Source: CAD feature listing. Evaluate the final solid. Frame: model axes, mm. A direction names the side the tool comes from. Give positions to 0.01 mm unless a question says otherwise; leave off trailing zeros. Loops run counter-clockwise (first coordinate to the right, second up) from the corner with the lowest first, then second, coordinate; pieces in that order, holes last. Notation, with made-up numbers: (42, 89.25) - (68, 89.25) arc R21 cw to (68, 128.25) - close; hole circle Ø4 at (88.5, 78.5). An arc over 180 degrees is marked (long way). Put each result on its own line as item: value.
```python
from build123d import *

# Parameters (mm, degrees)
SKETCH_1_W                = 90
SKETCH_1_H                = 150
EXTRUDE_1_DEPTH           = 5
SKETCH_4_R                = 36
CUT_EXTRUDE_1_DEPTH       = 89.034084308
HOLE_WIZARD_3_D           = 6.6
HOLE_WIZARD_3_CBORE_D     = 11
HOLE_WIZARD_3_CBORE_DEPTH = 6.8
HOLE_START                = -1.8
HOLE_WIZARD_2_DEPTH       = 6.8
HOLE_START_2              = -5
HOLE_WIZARD_2_2_DEPTH     = 3.2
CHAMFER_1_SIZE            = 12


# Read off the part's stored shape, not the designer's step: 打孔尺寸(%根据)内六角圆柱头螺钉的类型2
with BuildPart() as part:
    # 草图1 → 凸台-拉伸1 (new, symmetric)
    with BuildSketch(Plane.XY):
        Rectangle(SKETCH_1_W, SKETCH_1_H)
    extrude(amount=EXTRUDE_1_DEPTH, both=True)

    # 草图4 → 切除-拉伸1 (cut, through all)
    with BuildSketch(Plane.XY.offset(5)):
        Circle(SKETCH_4_R)
    extrude(amount=-CUT_EXTRUDE_1_DEPTH, mode=Mode.SUBTRACT)

    # 打孔尺寸(%根据)内六角圆柱头螺钉的类型3 (through all)
    with Locations(Plane(origin=(-31.75, 31.75, 5), x_dir=(1, 0, 0), z_dir=(0, 0, 1))):
        with Locations((0, 0), (63.5, 0), (0, -63.5), (63.5, -63.5)):
            CounterBoreHole(HOLE_WIZARD_3_D / 2, HOLE_WIZARD_3_CBORE_D / 2, HOLE_WIZARD_3_CBORE_DEPTH)

    # 打孔尺寸(%根据)内六角圆柱头螺钉的类型2 outline → 打孔尺寸(%根据)内六角圆柱头螺钉的类型2 (cut)
    with BuildSketch(Plane.XY.offset(HOLE_START)):
        with BuildLine():
            Line((-34, 59.5), (-26, 59.5))
            ThreePointArc((-26, 59.5), (-20.5, 65), (-26, 70.5))
            Line((-26, 70.5), (-34, 70.5))
            ThreePointArc((-34, 70.5), (-39.5, 65), (-34, 59.5))
        make_face()
        with BuildLine():
            ThreePointArc((34, 59.5), (39.5, 65), (34, 70.5))
            Line((34, 70.5), (26, 70.5))
            ThreePointArc((26, 70.5), (20.5, 65), (26, 59.5))
            Line((26, 59.5), (34, 59.5))
        make_face()
        with BuildLine():
            Line((-34, -70.5), (-26, -70.5))
            ThreePointArc((-26, -70.5), (-20.5, -65), (-26, -59.5))
            Line((-26, -59.5), (-34, -59.5))
            ThreePointArc((-34, -59.5), (-39.5, -65), (-34, -70.5))
        make_face()
        with BuildLine():
            ThreePointArc((34, -70.5), (39.5, -65), (34, -59.5))
            Line((34, -59.5), (26, -59.5))
            ThreePointArc((26, -59.5), (20.5, -65), (26, -70.5))
            Line((26, -70.5), (34, -70.5))
        make_face()
    extrude(amount=HOLE_WIZARD_2_DEPTH, mode=Mode.SUBTRACT)

    # Hole Wizard 2 2 outline → Hole Wizard 2 2 (cut)
    with BuildSketch(Plane.XY.offset(HOLE_START_2)):
        with BuildLine():
            Line((-34, 61.7), (-26, 61.7))
            ThreePointArc((-26, 61.7), (-22.7, 65), (-26, 68.3))
            Line((-26, 68.3), (-34, 68.3))
            ThreePointArc((-34, 68.3), (-37.3, 65), (-34, 61.7))
        make_face()
        with BuildLine():
            ThreePointArc((34, 61.7), (37.3, 65), (34, 68.3))
            Line((34, 68.3), (26, 68.3))
            ThreePointArc((26, 68.3), (22.7, 65), (26, 61.7))
            Line((26, 61.7), (34, 61.7))
        make_face()
        with BuildLine():
            Line((-34, -68.3), (-26, -68.3))
            ThreePointArc((-26, -68.3), (-22.7, -65), (-26, -61.7))
            Line((-26, -61.7), (-34, -61.7))
            ThreePointArc((-34, -61.7), (-37.3, -65), (-34, -68.3))
        make_face()
        with BuildLine():
            ThreePointArc((34, -68.3), (37.3, -65), (34, -61.7))
            Line((34, -61.7), (26, -61.7))
            ThreePointArc((26, -61.7), (22.7, -65), (26, -68.3))
            Line((26, -68.3), (34, -68.3))
        make_face()
    extrude(amount=HOLE_WIZARD_2_2_DEPTH, mode=Mode.SUBTRACT)

    # 倒角1
    chamfer_1_edges = [part.edges().sort_by_distance(p)[0] for p in [
        (45, -75, 0),
        (-45, -75, 0),
        (-45, 75, 0),
        (45, 75, 0),
    ]]
    chamfer(chamfer_1_edges, length=CHAMFER_1_SIZE)


solid = part.part
```
1) Mould query, pull axis X, two halves, no side actions, for faces 4 (the flat face through (19, -32, -5)), 5 (the cylindrical face through (31, 37.2, 1.6)). Classes: pulls with the +X half, pulls with the -X half, needs draft (parallel to the pull), parting line crosses it, or undercut.
Check result:
face 4: needs draft
face 5: undercut
2) Section query C-C, the plane z = -3.5. State how many separate pieces and enclosed holes the cut face has, plus the area to 3 significant figures.
Check result:
separate pieces: 1
enclosed holes: 9
area: 8,660 mm²
3) Section query A-A, the plane y = 0. Output: boundary loops of the cut face in (x, z), plus the area to 3 significant figures.
Check result:
outline: (-45, -5) - (-36, -5) - (-36, 5) - (-45, 5) - close; (36, -5) - (45, -5) - (45, 5) - (36, 5) - close
area: 180 mm²
4) Material intervals for line 1 along Y through (x, z) = (23, 2); line 2 along X through (y, z) = (-30, -2); line 3 along Y through (x, z) = (-23, -4), sorted ascending. Write a range as [from, to].
Check result:
line 1: [-75, -69.61], [-60.39, -27.69], [27.69, 60.39], [69.61, 75]
line 2: [-45, -34.55], [-28.95, -19.9], [19.9, 28.95], [34.55, 45]
line 3: [-75, -66.37], [-63.63, -27.69], [27.69, 63.63], [66.37, 75]
5) Section query B-B, the plane y = 65. Output: boundary loops of the cut face in (x, z).
Check result:
outline: (-43, -5) - (-37.3, -5) - (-37.3, -1.8) - (-39.5, -1.8) - (-39.5, 5) - (-43, 5) - close; (-22.7, -5) - (22.7, -5) - (22.7, -1.8) - (20.5, -1.8) - (20.5, 5) - (-20.5, 5) - (-20.5, -1.8) - (-22.7, -1.8) - close; (37.3, -5) - (43, -5) - (43, 5) - (39.5, 5) - (39.5, -1.8) - (37.3, -1.8) - close
6) Pin query (flat end, axial travel): P1, Ø5.5, axis at x = 28.5, y = 64, coming from the +Z side; P2, Ø12, axis at x = 31, y = -31, coming from the +Z side. Return the tip coordinate at first contact, or that it passes through.
Check result:
P1: z = -1.8
P2: z = 5
7) Section query D-D, the plane x = 24.5. Output: boundary loops of the cut face in (y, z), plus the area to 3 significant figures.
Check result:
outline: (-75, -5) - (-67.94, -5) - (-67.94, -1.8) - (-70.29, -1.8) - (-70.29, 5) - (-75, 5) - close; (-62.06, -5) - (-26.38, -5) - (-26.38, 5) - (-59.71, 5) - (-59.71, -1.8) - (-62.06, -1.8) - close; (26.38, -5) - (62.06, -5) - (62.06, -1.8) - (59.71, -1.8) - (59.71, 5) - (26.38, 5) - close; (67.94, -5) - (75, -5) - (75, 5) - (70.29, 5) - (70.29, -1.8) - (67.94, -1.8) - close
area: 791 mm²
8) Access query for faces 1 (the flat face through (19, 34, 5)), 2 (the cylindrical face through (26.255, -31.508, 1.648)), 3 (the cylindrical face through (-22.7, 64.9, -3.4)). Directions: +Z, -Z, +X, -X, +Y, -Y. A direction counts if a zero-diameter tool reaches every point of the face in a straight line with its end or side. Return the directions, or none.
Check result:
face 1: +Z, +X, -X, +Y, -Y
face 2: +Z
face 3: +Z, -Z
